Autodesk Inventor part; units mm, degrees
ref_plane "YZ Plane" through (0, 0, 0) normal (1, 0, 0) x (0, 1, 0)
ref_plane "XZ Plane" through (0, 0, 0) normal (0, 1, 0) x (-1, 0, 0)
ref_plane "XY Plane" through (0, 0, 0) normal (0, 0, 1) x (1, 0, 0)
ref_plane "Work Plane1" through (-1022, 1522, 0) normal (0, 0, 1) x (1, 0, 0)
sketch "Sketch1" plane through (-1022, 1522, 0) normal (0, 0, 1) x (1, 0, 0)
  line L0 (1022, 22) -> (1022, -1522)
  line L1 (1022, 22) -> (1000, 22)
  line L2 (1000, -1522) -> (1000, 22)
  line L3 (1022, -1522) -> (1000, -1522)
  circle A0 centre (880.1401, -150.1401) radius 55
  line L4 (0, 0) -> (1000, 0)
  line L5 (1000, 0) -> (1000, 22)
  line L6 (0, 22) -> (1000, 22)
  line L7 (0, 0) -> (0, 22)
  line L8 (752, 0) -> (752, -300)
  line L9 (752, -300) -> (1022, -300)
  line L10 (1022, -300) -> (1022, -232)
  line L11 (1022, -232) -> (820, -232)
  line L12 (820, -232) -> (820, 0)
  line L13 (1022, 22) -> (1000, 22)
  line L14 (820, 0) -> (752, 0)
  line L15 (0, 0) -> (2000, 0) construction
  line L16 (0, 0) -> (2000, 0) construction
  point P0 (1022, -1522)
  dimension "d0" = 270
  dimension "d1" = 300
  dimension "d3" = 232
  dimension "d4" = 202
  dimension "d6" = 2000
  dimension "d8" = 1022
extrude "Extrusion1" add sketch "Sketch1" along normal blind 22 contours L0 L9 L2 L11 | L2 L9 L8 L4 L12 L11
properties part number "Jig_nodeAirInlet"
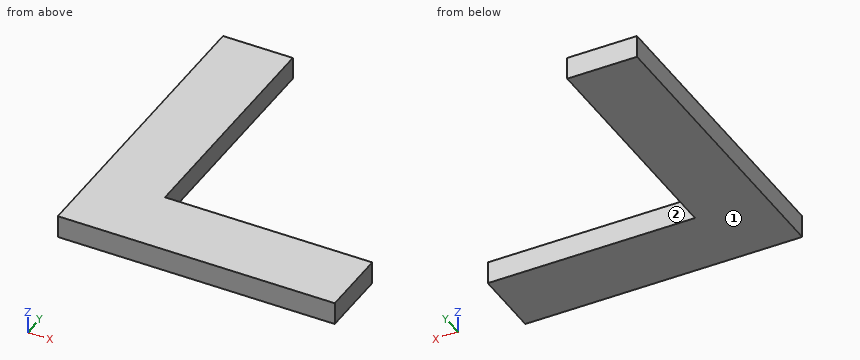
Verification items for the finished model (mm, model axes). Face numbers are marked on the shaded views. A direction names the side the tool comes from. Round coordinates to 2 decimals unless told otherwise and drop trailing zeros. Loops run counter-clockwise (first coordinate to the right, second up) from the corner with the lowest first, then second, coordinate; pieces in that order, holes last. Notation, with made-up numbers: (89, 26.5) - (108, 26.5) arc R13 ccw to (108, 48.5) - close; hole circle Ø7 at (-19, 31.25). An arc over 180 degrees is marked (long way). Use one line per item in the form item = value.
1. Section check A-A on z = 9.5. Record the cut outline in (x, y).
A:
outline = (-270, 1222) - (0, 1222) - (0, 1290) - (-202, 1290) - (-202, 1522) - (-270, 1522) - close
2. Scan lines: probe 1 along Y at (x, z) = (-127.5, 11); probe 2 along X at (y, z) = (1479, 18.5). Record each from-to range of solid material in increasing order.
A:
probe_1 = 1222 to 1290
probe_2 = -270 to -202
3. Section check C-C on y = 1486.5. Record the cut outline in (x, z), and give its area (3 significant figures).
A:
outline = (-270, 0) - (-202, 0) - (-202, 22) - (-270, 22) - close
area = 1,500 mm²
4. Gauge pin test, flat ends, axial feed: pin 1 Ø1 at (x, z) = (-112, 7.5) entering from +Y; pin 2 Ø11 at (y, z) = (1448, 9) entering from +X. Record the tip position at first contact, or that the pin passes through.
A:
pin_1 = 1290
pin_2 = -202
5. Section check B-B on x = -68. Record the cut outline in (y, z), and give its area (3 significant figures).
A:
outline = (1222, 0) - (1290, 0) - (1290, 22) - (1222, 22) - close
area = 1,500 mm²
6. Access from +Z, -Z, +X, -X, +Y, -Y to the whole of each face (thin tool, end or side, straight path). Record for the marked faces 1 and 2.
A:
face_1 = -Z, +X, -X, +Y, -Y
face_2 = +Z, -Z, +X, +Y
